```python
from build123d import *

# Parameters (mm, degrees)
SKETCH1_W                = 40
SKETCH1_H                = 40
SKETCH1_R                = 2.375
BOSS_EXTRUDE1_DEPTH      = 40
CUT_EXTRUDE1_DEPTH       = 61
CUT_EXTRUDE1_DEPTH_BACK  = 61
CUT_EXTRUDE2_DEPTH       = 49.989795019
CUT_EXTRUDE2_DEPTH_BACK  = 35
SKETCH6_W                = 30
SKETCH6_H                = 35
SKETCH3_R                = 3
CUT_EXTRUDE3_DEPTH       = 61
BOSS_EXTRUDE2_DEPTH      = 30
SKETCH8_R                = 1.8
CUT_EXTRUDE4_DEPTH       = 68.082039325
BOSS_EXTRUDE4_START      = -35
SKETCH10_W               = 5
SKETCH10_H               = 35
BOSS_EXTRUDE4_DEPTH      = 115
SKETCH11_R               = 2.375
CUT_EXTRUDE5_DEPTH       = 70
CUT_EXTRUDE6_DEPTH       = 115.891252931
CUT_EXTRUDE6_DEPTH_BACK  = 115.891252931
SKETCH14_W               = 30
SKETCH14_H               = 3
BOSS_EXTRUDE10_DEPTH     = 35
CUT_EXTRUDE7_DEPTH       = 108.819293264
CUT_EXTRUDE7_DEPTH_BACK  = 1.5
SKETCH16_W               = 30
SKETCH16_H               = 34
CUT_EXTRUDE8_DEPTH       = 32
CUT_EXTRUDE8_DEPTH_BACK  = 32.5
CUT_EXTRUDE9_DEPTH       = 115.04494728
CUT_EXTRUDE9_DEPTH_BACK  = 115.04494728
SKETCH19_R               = 1.8
SKETCH3_2_R              = 3
BOSS_EXTRUDE11_DEPTH     = 5
SKETCH20_W               = 30
SKETCH20_H               = 35
CUT_EXTRUDE10_DEPTH      = 10
CUT_EXTRUDE11_DEPTH      = 110.544511501
CUT_EXTRUDE11_DEPTH_BACK = 110.544511501
SKETCH22_R               = 3
SKETCH21_R               = 2.375
BOSS_EXTRUDE13_DEPTH     = 3.5
CUT_EXTRUDE12_DEPTH      = 110.544511501
CUT_EXTRUDE12_DEPTH_BACK = 110.544511501
SKETCH23_R               = 0.815
CUT_EXTRUDE13_DEPTH      = 109.315511355
CUT_EXTRUDE13_DEPTH_BACK = 1.5
SKETCH24_R               = 12.5
CUT_EXTRUDE14_DEPTH      = 17.5
CUT_EXTRUDE14_DEPTH_BACK = 17.5


with BuildPart() as part:
    # Sketch1 → Boss-Extrude1 (new body)
    with BuildSketch(Plane(origin=(0, 0, 0), x_dir=(1, 0, 0), z_dir=(0, 1, 0))):
        Rectangle(SKETCH1_W, SKETCH1_H)
        with Locations(Location((6.88, 0, 0), (0, 0, 270))):
            Circle(SKETCH1_R, mode=Mode.SUBTRACT)
        with Locations(Location((-0.009652089, -6.889652089, 0), (0, 0, 270))):
            Circle(SKETCH1_R, mode=Mode.SUBTRACT)
        with Locations(Location((-6.899304178, 0, 0), (0, 0, 270))):
            Circle(SKETCH1_R, mode=Mode.SUBTRACT)
        with Locations(Location((-0.009652089, 6.889652089, 0), (0, 0, 270))):
            Circle(SKETCH1_R, mode=Mode.SUBTRACT)
    extrude(amount=BOSS_EXTRUDE1_DEPTH)

    # Sketch4 → Cut-Extrude1 (cut, two sides: drawn at the far end of the back side and taken through both)
    with BuildSketch(Plane.ZY.offset(20).offset(-CUT_EXTRUDE1_DEPTH_BACK)):
        with BuildLine():
            Line((-20, 35), (-20, 0))
            Line((-20, 0), (15, 0))
            ThreePointArc((15, 0), (4.748737342, 24.748737342), (-20, 35))
        make_face()
    extrude(amount=CUT_EXTRUDE1_DEPTH + CUT_EXTRUDE1_DEPTH_BACK, mode=Mode.SUBTRACT)

    # Sketch6 → Cut-Extrude2 (cut, two sides: drawn at the far end of the back side and taken through both)
    with BuildSketch(Plane.XZ.offset(-CUT_EXTRUDE2_DEPTH_BACK)):
        with Locations((0, -2.5)):
            Rectangle(SKETCH6_W, SKETCH6_H)
    extrude(amount=CUT_EXTRUDE2_DEPTH + CUT_EXTRUDE2_DEPTH_BACK, mode=Mode.SUBTRACT)

    # Sketch3 → Cut-Extrude3 (cut, through all)
    with BuildSketch(Plane.XY.offset(20)):
        with Locations((0, 13)):
            Circle(SKETCH3_R)
        with Locations((-7, 20)):
            Circle(SKETCH3_R)
        with Locations((7, 20)):
            Circle(SKETCH3_R)
    extrude(amount=-CUT_EXTRUDE3_DEPTH, mode=Mode.SUBTRACT)

    # Sketch7 → Boss-Extrude2 (add)
    with BuildSketch(Plane.XY.offset(20)):
        Polygon((-17.5, 40), (17.5, 40), (17.5, 5), (12.5, 5), (12.5, 30), (-12.5, 30), (-12.5, 5), (-17.5, 5), (-17.5, 23.79079138), align=None)
    extrude(amount=BOSS_EXTRUDE2_DEPTH)

    # Sketch8 → Cut-Extrude4 (cut, through all)
    with BuildSketch(Plane(origin=(0, 40, 0), x_dir=(1, 0, 0), z_dir=(0, 1, 0))):
        with Locations(Location((5, -32.5, 0), (0, 0, 270))):
            Circle(SKETCH8_R)
        with Locations(Location((-5, -32.5, 0), (0, 0, 270))):
            Circle(SKETCH8_R)
    extrude(amount=-CUT_EXTRUDE4_DEPTH, mode=Mode.SUBTRACT)

    # Sketch10 → Boss-Extrude4 (add)
    with BuildSketch(Plane(origin=(0, 0, -20), x_dir=(-1, 0, 0), z_dir=(0, 0, -1)).offset(BOSS_EXTRUDE4_START)):
        Polygon((20, 40), (-20, 40), (-20, 35), (-15, 35), (15, 35), (20, 35), align=None)
        with Locations((17.5, 17.5)):
            Rectangle(SKETCH10_W, SKETCH10_H)
        with Locations((-17.5, 17.5)):
            Rectangle(SKETCH10_W, SKETCH10_H)
    extrude(amount=BOSS_EXTRUDE4_DEPTH)

    # Sketch11 → Cut-Extrude5 (cut)
    with BuildSketch(Plane(origin=(0, 40, 0), x_dir=(1, 0, 0), z_dir=(0, 1, 0))):
        with Locations(Location((-0.009652089, -6.889652089, 0), (0, 0, 270))):
            Circle(SKETCH11_R)
        with Locations(Location((6.88, 0, 0), (0, 0, 270))):
            Circle(SKETCH11_R)
        with Locations(Location((-0.009652089, 6.889652089, 0), (0, 0, 270))):
            Circle(SKETCH11_R)
        with Locations(Location((-6.899304178, 0, 0), (0, 0, 270))):
            Circle(SKETCH11_R)
    extrude(amount=-CUT_EXTRUDE5_DEPTH, mode=Mode.SUBTRACT)

    # Sketch13 → Cut-Extrude6 (cut, two sides: drawn at the far end of the back side and taken through both)
    with BuildSketch(Plane.ZY.offset(20).offset(-CUT_EXTRUDE6_DEPTH_BACK)):
        with BuildLine():
            Line((-86.5, 26.8), (-83.5, 26.8))
            ThreePointArc((-83.5, 26.8), (-81.7, 25), (-83.5, 23.2))
            Line((-83.5, 23.2), (-86.5, 23.2))
            ThreePointArc((-86.5, 23.2), (-88.3, 25), (-86.5, 26.8))
        make_face()
        with BuildLine():
            Line((-86.5, 8.2), (-83.5, 8.2))
            ThreePointArc((-83.5, 8.2), (-81.7, 10), (-83.5, 11.8))
            Line((-83.5, 11.8), (-86.5, 11.8))
            ThreePointArc((-86.5, 11.8), (-88.3, 10), (-86.5, 8.2))
        make_face()
    extrude(amount=CUT_EXTRUDE6_DEPTH + CUT_EXTRUDE6_DEPTH_BACK, mode=Mode.SUBTRACT)

    # Sketch14 → Boss-Extrude10 (add)
    with BuildSketch(Plane.XZ.offset(-35)):
        with Locations((0, -98.5)):
            Rectangle(SKETCH14_W, SKETCH14_H)
        with Locations((0, -45.5)):
            Rectangle(SKETCH14_W, SKETCH14_H)
        with Locations((0, -20.5)):
            Rectangle(SKETCH14_W, SKETCH14_H)
        with Locations((0, -68.5)):
            Rectangle(SKETCH14_W, SKETCH14_H)
    extrude(amount=BOSS_EXTRUDE10_DEPTH)

    # Sketch16 → Cut-Extrude7 (cut, two sides: drawn at the far end of the back side and taken through both)
    with BuildSketch(Plane.XZ.offset(-35).offset(-CUT_EXTRUDE7_DEPTH_BACK)):
        with Locations((0, -2)):
            Rectangle(SKETCH16_W, SKETCH16_H)
    extrude(amount=CUT_EXTRUDE7_DEPTH + CUT_EXTRUDE7_DEPTH_BACK, mode=Mode.SUBTRACT)

    # Sketch17 → Cut-Extrude8 (cut, two sides: drawn at the far end of the back side and taken through both)
    with BuildSketch(Plane(origin=(0, 0, -47), x_dir=(-1, 0, 0), z_dir=(0, 0, -1)).offset(-CUT_EXTRUDE8_DEPTH_BACK)):
        with BuildLine():
            Line((-15, -8.523755025), (-15, 5.476244975))
            ThreePointArc((-15, 5.476244975), (0, 20.476244975), (15, 5.476244975))
            Line((15, 5.476244975), (15, -8.523755025))
            ThreePointArc((15, -8.523755025), (0, -23.523755025), (-15, -8.523755025))
        make_face()
    extrude(amount=CUT_EXTRUDE8_DEPTH + CUT_EXTRUDE8_DEPTH_BACK, mode=Mode.SUBTRACT)

    # Sketch19 → Cut-Extrude9 (cut, two sides: drawn at the far end of the back side and taken through both)
    with BuildSketch(Plane.ZY.offset(17.5).offset(-CUT_EXTRUDE9_DEPTH_BACK)):
        with Locations(Location((40, 17.5, 0), (0, 0, 270))):
            Circle(SKETCH19_R)
    extrude(amount=CUT_EXTRUDE9_DEPTH + CUT_EXTRUDE9_DEPTH_BACK, mode=Mode.SUBTRACT)

    # Sketch3<2> → Boss-Extrude11 (add)
    with BuildSketch(Plane.XY.offset(20)):
        with Locations((0, 13)):
            Circle(SKETCH3_2_R)
        with Locations((-7, 20)):
            Circle(SKETCH3_2_R)
        with Locations((7, 20)):
            Circle(SKETCH3_2_R)
    extrude(amount=-BOSS_EXTRUDE11_DEPTH)

    # Sketch20 → Cut-Extrude10 (cut)
    with BuildSketch(Plane.XY.offset(-97)):
        with Locations((0, 17.5)):
            Rectangle(SKETCH20_W, SKETCH20_H)
    extrude(amount=-CUT_EXTRUDE10_DEPTH, mode=Mode.SUBTRACT)

    # Sketch22 → Cut-Extrude11 (cut, two sides: drawn at the far end of the back side and taken through both)
    with BuildSketch(Plane(origin=(0, 40, 0), x_dir=(1, 0, 0), z_dir=(0, 1, 0)).offset(-CUT_EXTRUDE11_DEPTH_BACK)):
        with Locations(Location((0, 0, 0), (0, 0, 270))):
            Circle(SKETCH22_R)
    extrude(amount=CUT_EXTRUDE11_DEPTH + CUT_EXTRUDE11_DEPTH_BACK, mode=Mode.SUBTRACT)

    # Sketch21 → Boss-Extrude13 (add)
    with BuildSketch(Plane(origin=(0, 40, 0), x_dir=(1, 0, 0), z_dir=(0, 1, 0))):
        with Locations((-0.009652089, -6.889652089)):
            Circle(SKETCH21_R)
        with Locations((6.88, 0)):
            Circle(SKETCH21_R)
        with Locations((-0.009652089, 6.889652089)):
            Circle(SKETCH21_R)
        with Locations((-6.899304178, 0)):
            Circle(SKETCH21_R)
    extrude(amount=-BOSS_EXTRUDE13_DEPTH)

    # Sketch23 → Cut-Extrude12 (cut, two sides: drawn at the far end of the back side and taken through both)
    with BuildSketch(Plane(origin=(0, 40, 0), x_dir=(1, 0, 0), z_dir=(0, 1, 0)).offset(-CUT_EXTRUDE12_DEPTH_BACK)):
        with Locations(Location((-5.656854249, 5.656854249, 0), (0, 0, 270))):
            Circle(SKETCH23_R)
        with Locations(Location((4.242640687, 4.242640687, 0), (0, 0, 270))):
            Circle(SKETCH23_R)
        with Locations(Location((5.656854249, -5.656854249, 0), (0, 0, 270))):
            Circle(SKETCH23_R)
        with Locations(Location((-4.242640687, -4.242640687, 0), (0, 0, 270))):
            Circle(SKETCH23_R)
    extrude(amount=CUT_EXTRUDE12_DEPTH + CUT_EXTRUDE12_DEPTH_BACK, mode=Mode.SUBTRACT)

    # Sketch24 → Cut-Extrude13 (cut, two sides: drawn at the far end of the back side and taken through both)
    with BuildSketch(Plane.XZ.offset(-36.5).offset(-CUT_EXTRUDE13_DEPTH_BACK)):
        with Locations(Location((0, 0, 0), (0, 0, 90))):
            Circle(SKETCH24_R)
    extrude(amount=CUT_EXTRUDE13_DEPTH + CUT_EXTRUDE13_DEPTH_BACK, mode=Mode.SUBTRACT)

    # Sketch25 → Cut-Extrude14 (cut, two sides: drawn at the far end of the back side and taken through both)
    with BuildSketch(Plane(origin=(0, 0, 0), x_dir=(0, 0, -1), z_dir=(1, 0, 0)).offset(-CUT_EXTRUDE14_DEPTH_BACK)):
        with BuildLine():
            Line((92.5, 25), (92.5, -7.922367103))
            ThreePointArc((92.5, -7.922367103), (85, -15.422367103), (77.5, -7.922367103))
            Line((77.5, -7.922367103), (77.5, 25))
            ThreePointArc((77.5, 25), (85, 32.5), (92.5, 25))
        make_face()
    extrude(amount=CUT_EXTRUDE14_DEPTH + CUT_EXTRUDE14_DEPTH_BACK, mode=Mode.SUBTRACT)


solid = part.part
```
Read the model definition and answer for the solid it produces. Units are mm, in the model's axes. A direction names the side the tool comes from. Coordinates: 2 decimals unless noted, no trailing zeros. Loops run counter-clockwise (first coordinate to the right, second up) from the corner with the lowest first, then second, coordinate; pieces in that order, holes last. Notation, with made-up numbers: (-36, -17.75) -> (14, -17.75) arc R25 cw to (14, 15.25) -> close; hole circle Ø7 at (-18, 65). An arc over 180 degrees is marked (long way). Return JSON: item names as keys, results as strings.
Item 1: Flat-ended cylindrical pins translate along their axes: P1, Ø4, axis at x = 12.5, y = 16, coming from the -Z side; P2, Ø20, axis at y = 17, z = 36, coming from the -X side; P3, Ø5.5, axis at x = 0, z = 0, coming from the -Y side; P4, Ø2, axis at x = 6, z = 23, coming from the -Y side. Find the tip coordinate at first contact, or state that the pin passes through.
Answers:
{"P1": "stops at z = -70", "P2": "stops at x = -17.5", "P3": "passes through", "P4": "stops at y = 30"}
Item 2: For a pull along Y with two mould halves and no side action, classify faces 3 (the cylindrical face through (18.8, 10, -81.7)), 4 (the flat face through (0, 40, -26)), 5 (the flat face through (0, 27, -70)) as +Y half, -Y half, draft (parallel to the pull), parting line (faces both ways), or undercut.
Answers:
{"face 3": "undercut", "face 4": "+Y half", "face 5": "draft"}
Item 3: Find section C-C (y = 9.5). Count the separate pieces of the cut face and the enclosed holes in it, plus the area to 3 significant figures.
Answers:
{"separate pieces": "3", "enclosed holes": "0", "area": "1,550 mm2"}
Item 4: Find section A-A (z = 0). Determine the outline of the cut face in (x, y).
Answers:
{"outline": "(-20, 0) -> (-15, 0) -> (-15, 36.5) -> (-12.5, 36.5) -> (-12.5, 38) -> (-3, 38) -> (-3, 40) -> (-20, 40) -> close; (3, 38) -> (12.5, 38) -> (12.5, 36.5) -> (15, 36.5) -> (15, 0) -> (20, 0) -> (20, 40) -> (3, 40) -> close"}
Item 5: Find section B-B (z = 32.5). Determine the outline of the cut face in (x, y).
Answers:
{"outline": "(-17.5, 5) -> (-12.5, 5) -> (-12.5, 30) -> (-6.8, 30) -> (-6.8, 40) -> (-17.5, 40) -> close; (-3.2, 30) -> (3.2, 30) -> (3.2, 40) -> (-3.2, 40) -> close; (6.8, 30) -> (12.5, 30) -> (12.5, 5) -> (17.5, 5) -> (17.5, 40) -> (6.8, 40) -> close"}
Item 6: For faces 1 (the flat face through (19, 11.8, -85)), 2 (the flat face through (0, 27, -44)), determine the directions among +Z, -Z, +X, -X, +Y, -Y from which every point of the face is accessible in a straight line to the end or side of a thin tool.
Answers:
{"face 1": "+X, -X", "face 2": "-Y"}
Item 7: Find the intervals of material crossed by probe 1 along Z at (x, y) = (14, 28); probe 2 along Z at (x, y) = (-9, 22.5); probe 3 along X at (y, z) = (24, 23), in increasing order.
Answers:
{"probe 1": "z = -70 to -67, -47 to -44, -22 to -19, 15 to 50", "probe 2": "z = -70 to -67, -47 to -44, -22 to -19, 15 to 20", "probe 3": "x = -17.5 to -12.5, 12.5 to 17.5"}
